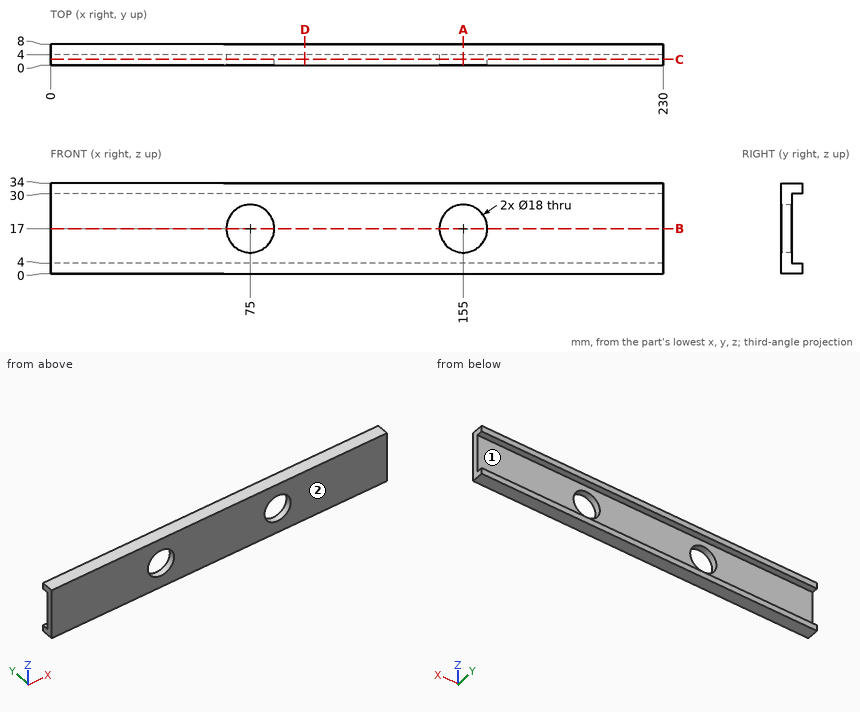
Geometry check sheet. Reference: drawing and pictorial views, mm from the part's lowest x, y, z. Give positions to 0.01 mm unless a question says otherwise; leave off trailing zeros. Loops run counter-clockwise (first coordinate to the right, second up) from the corner with the lowest first, then second, coordinate; pieces in that order, holes last.
1. Section check C-C, the plane y = 2.25. Enter the section's corners in (x, z), then the cut area to 3 significant figures.
2. Section check A-A, the plane x = 155. Enter the section's corners in (y, z).
3. Thickness scan on line 1 (Z direction, x = 25.5, y = 5); line 2 (Z direction, x = 75, y = 1.75); line 3 (X direction, y = 3, z = 21). Record the ranges inside material, lowest first.
4. Section check B-B, the plane z = 17. Enter the section's corners in (x, y).
5. Go/stop test with a flat-tipped pin: pin 1 Ø4 at (x, z) = (125, 27) entering from +Y. Record where the tip stops, or that it passes through.
6. Section check D-D, the plane x = 95.5. Enter the section's corners in (y, z), then the cut area to 3 significant figures.
7. Mould release check, pull along Z, two halves, no side actions. Record for the marked faces 1 and 2: released by +Z, released by -Z, zero draft, split by the parting line, or undercut.
Geometry says:
1. outline: (0, 0) - (230, 0) - (230, 34) - (0, 34) - close; hole circle Ø18 at (75, 17); hole circle Ø18 at (155, 17)
1. area: 7,310 mm2
2. outline: (0, 0) - (8, 0) - (8, 4) - (4, 4) - (4, 8) - (0, 8) - close; (0, 26) - (4, 26) - (4, 30) - (8, 30) - (8, 34) - (0, 34) - close
3. line 1: z = 0 to 4, 30 to 34
3. line 2: z = 0 to 8, 26 to 34
3. line 3: x = 0 to 66.94, 83.06 to 146.94, 163.06 to 230
4. outline: (0, 0) - (66, 0) - (66, 4) - (0, 4) - close; (84, 0) - (146, 0) - (146, 4) - (84, 4) - close; (164, 0) - (230, 0) - (230, 4) - (164, 4) - close
5. pin 1: stops at y = 4
6. outline: (0, 0) - (8, 0) - (8, 4) - (4, 4) - (4, 30) - (8, 30) - (8, 34) - (0, 34) - close
6. area: 168 mm2
7. face 1: undercut
7. face 2: zero draft
